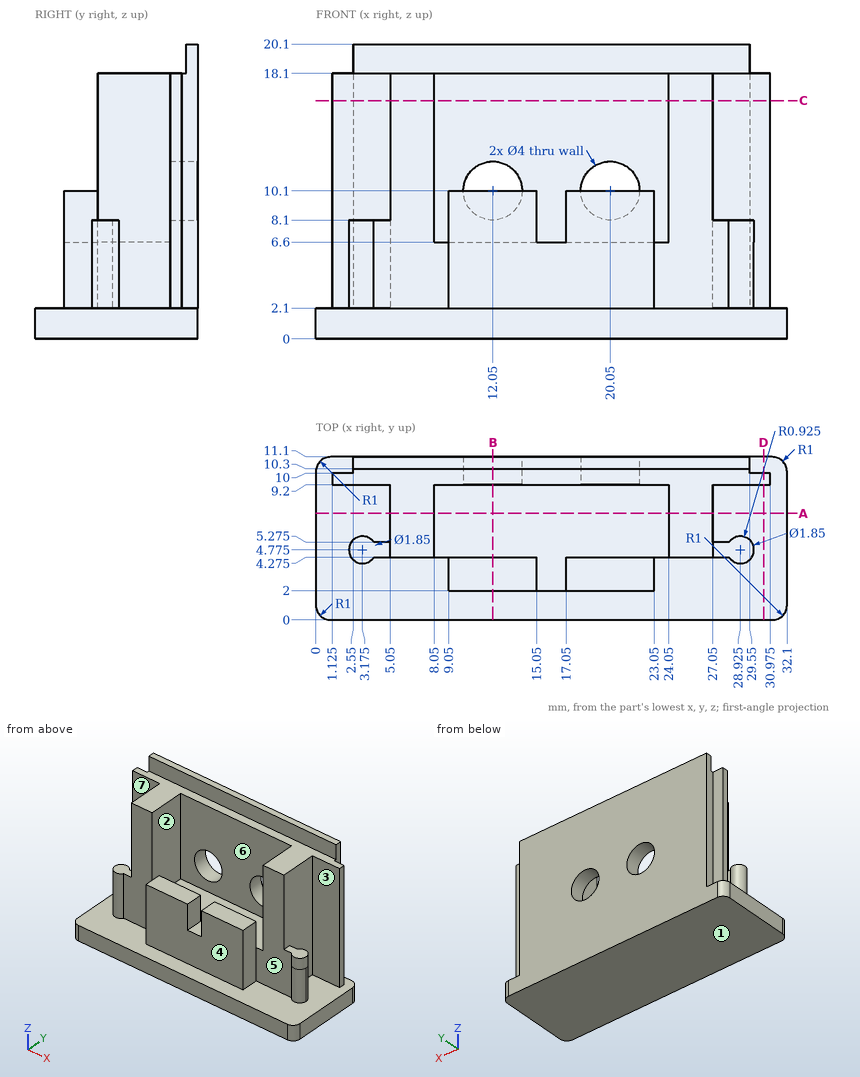
Verification items for this drawing (mm, ordinates from the low corner). A direction names the side the tool comes from. Give positions to 0.01 mm unless a question says otherwise; leave off trailing zeros. Loops run counter-clockwise (first coordinate to the right, second up) from the corner with the lowest first, then second, coordinate; pieces in that order, holes last.
1. Cross-section at C-C on z = 16.25. Record the cut outline in (x, y) (3 decimals).
Derived:
outline: (1.125, 9.2) - (5.05, 9.2) - (5.05, 4.275) - (8.05, 4.275) - (8.05, 9.2) - (24.05, 9.2) - (24.05, 4.275) - (27.05, 4.275) - (27.05, 9.2) - (30.975, 9.2) - (30.975, 10) - (29.55, 10) - (29.55, 11.1) - (2.55, 11.1) - (2.55, 10) - (1.125, 10) - close
2. Tool access check on the marked faces 3, 4, 5, 6 and 7. Record the directions out of +Z, -Z, +X, -X, +Y, -Y that give a thin tool (end or side, any length) a straight path to the whole face; none if there is none.
Derived:
face 3: +Z, +X
face 4: +Z, +X, -X, -Y
face 5: +Z, -Y
face 6: +Z
face 7: +Z, -X
3. Cross-section at D-D on x = 30.5. Record the cut outline in (y, z).
Derived:
outline: (0, 0) - (11.1, 0) - (11.1, 2.1) - (10, 2.1) - (10, 18.1) - (9.2, 18.1) - (9.2, 2.1) - (0, 2.1) - close
4. Cross-section at B-B on x = 12.05. Record the cut outline in (y, z) (3 decimals).
Derived:
outline: (0, 0) - (11.1, 0) - (11.1, 8.1) - (9.2, 8.1) - (9.2, 6.6) - (4.275, 6.6) - (4.275, 10.1) - (2, 10.1) - (2, 2.1) - (0, 2.1) - close; (9.2, 12.1) - (11.1, 12.1) - (11.1, 20.1) - (10.3, 20.1) - (10.3, 18.1) - (9.2, 18.1) - close
5. Release check for a two-part mould opening along X. For the marked faces 1 and 2 record: +X half, -X half, draft (parallel to the pull), parting line (faces both ways), or undercut.
Derived:
face 1: draft
face 2: undercut
6. Material ranges on probe 1 along X at (y, z) = (8.25, 16); probe 2 along Z at (x, y) = (12.05, 10.4); probe 3 along Y at (x, z) = (18, 18.5), recorded low to high.
Derived:
probe 1: x = 5.05 to 8.05, 24.05 to 27.05
probe 2: z = 0 to 8.1, 12.1 to 20.1
probe 3: y = 10.3 to 11.1
7. Cross-section at A-A on y = 7.25. Record the cut outline in (x, z), and give its area (3 significant figures).
Derived:
outline: (0, 0) - (32.1, 0) - (32.1, 2.1) - (27.05, 2.1) - (27.05, 18.1) - (24.05, 18.1) - (24.05, 6.6) - (8.05, 6.6) - (8.05, 18.1) - (5.05, 18.1) - (5.05, 2.1) - (0, 2.1) - close
area: 235 mm2
8. Go/stop test with flat-tipped pins: P1, Ø0.9, axis at y = 9.5, z = 11.5, coming from the -X side (3 decimals); P2, Ø2, axis at y = 1.5, z = 7.5, coming from the -X side; P3, Ø2.5, axis at x = 12, y = 2.5, coming from the +Z side. Record where each tip stops, or that it passes through.
Derived:
P1: stops at x = 1.125
P2: stops at x = 9.05
P3: stops at z = 10.1
